Here's how the part is built. I have some questions about the finished solid (model axes, mm). Face numbers are marked on the shaded views. A direction names the side the tool comes from. Give positions to 0.01 mm unless a question says otherwise; leave off trailing zeros. Loops run counter-clockwise (first coordinate to the right, second up) from the corner with the lowest first, then second, coordinate; pieces in that order, holes last. Notation, with made-up numbers: (76, 43.5) - (87, 43.5) arc R10 ccw to (87, 49.5) - close; hole circle Ø3 at (-24, -22.5). An arc over 180 degrees is marked (long way). Return JSON: item names as keys, results as strings. Group by question number.
(1) On a 3-axis mill with a long thin cutter (end or side, diameter ignored), from which of +Z, -Z, +X, -X, +Y, -Y can I reach the whole of each face in a straight line? I mean the marked faces 1 and 2. Say none if no direction works.
(2) If we section it at A-A (z = -3.25): Please give me the cut outline in (x, y), then the cut area to 3 significant figures.
(3) If we mould it in two halves opening along Y, with no side actions, what happens to the marked faces 3, 4, 5 and 6? For each: released by +Y, released by -Y, zero draft, split by the parting line, or undercut.
(4) If we section it at B-B (y = -4): Please give me the cut outline in (x, z).
(5) If we section it at C-C (x = 17): Please give me the cut outline in (y, z), then the cut area to 3 significant figures.
(6) I need wall thicknesses on probe 1 along Z at (x, y) = (0, -5.75); probe 2 along Y at (x, z) = (17, 8); probe 3 along X at (y, z) = (-4.75, -7.5). Which ranges of each line are inside material? Lowest first, please. Write a range as [from, to].
(7) If we section it at D-D (z = 7.5): Please give me the cut outline in (x, y), then the cut area to 3 significant figures.
(8) For P1, Ø5, axis at x = -16.5, z = -7.5, coming from the +Y side; P2, Ø4, axis at x = -4.5, y = -4.5, coming from the -Z side, each with a flat end and sliding along its axis, tell me the tip position at first contact or that it passes through.
```python
from build123d import *

# Parameters (mm, degrees)
F0_R     = 3
F0_R_2   = 4
F1_DEPTH = 8
F2_R     = 2.25
F3_DEPTH = 28.001


with BuildPart() as f1:
    # F0 (on Front) → F1 (new body)
    with BuildSketch(Plane.XZ):
        Polygon((21, 14), (-21, 14), (-21, -14), (-13, -14), (-13, -2), (13, -2), (13, -14), (21, -14), align=None)
        with Locations((-10, 9)):
            Circle(F0_R, mode=Mode.SUBTRACT)
        with Locations((0, 7)):
            Circle(F0_R_2, mode=Mode.SUBTRACT)
        with Locations((10, 9)):
            Circle(F0_R, mode=Mode.SUBTRACT)
    extrude(amount=F1_DEPTH)

    # F2 (on face) → F3 (cut, through all)
    with BuildSketch(Plane.XY.offset(14)):
        with Locations((-17, -4)):
            Circle(F2_R)
        with Locations((17, -4)):
            Circle(F2_R)
    extrude(amount=-F3_DEPTH, mode=Mode.SUBTRACT)


solid = f1.part
```
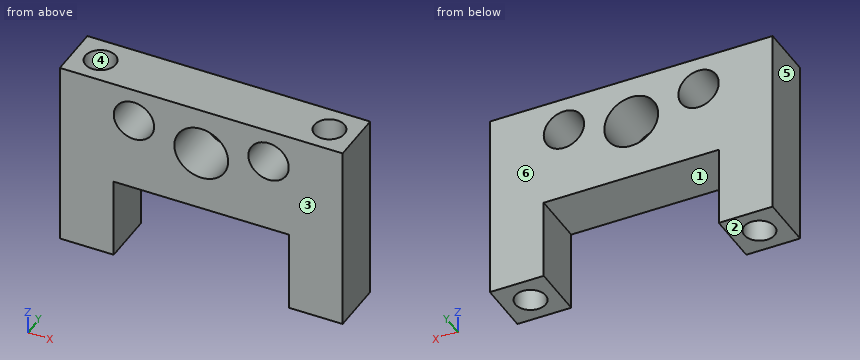
Values:
{
 "1": {"face 1": "-Z, +Y, -Y", "face 2": "-Z, +X, -X, +Y, -Y"},
 "2": {"outline": "(-21, -8) - (-13, -8) - (-13, 0) - (-21, 0) - close; (13, -8) - (21, -8) - (21, 0) - (13, 0) - close; hole circle Ø4.5 at (-17, -4); hole circle Ø4.5 at (17, -4)", "area": "96.2 mm2"},
 "3": {"face 3": "released by -Y", "face 4": "undercut", "face 5": "zero draft", "face 6": "released by +Y"},
 "4": {"outline": "(-21, -14) - (-19.25, -14) - (-19.25, 14) - (-21, 14) - close; (-14.75, -14) - (-13, -14) - (-13, -2) - (13, -2) - (13, -14) - (14.75, -14) - (14.75, 14) - (-14.75, 14) - close; (19.25, -14) - (21, -14) - (21, 14) - (19.25, 14) - close; hole circle Ø6 at (-10, 9); hole circle Ø8 at (0, 7); hole circle Ø6 at (10, 9)"},
 "5": {"outline": "(-8, -14) - (-6.25, -14) - (-6.25, 14) - (-8, 14) - close; (-1.75, -14) - (0, -14) - (0, 14) - (-1.75, 14) - close", "area": "98.0 mm2"},
 "6": {"probe 1": "[-2, 3], [11, 14]", "probe 2": "[-8, -6.25], [-1.75, 0]", "probe 3": "[-21, -19.12], [-14.88, -13], [13, 14.88], [19.12, 21]"},
 "7": {"outline": "(-21, -8) - (-12.6, -8) - (-12.6, 0) - (-21, 0) - close; (-7.4, -8) - (-3.97, -8) - (-3.97, 0) - (-7.4, 0) - close; (3.97, -8) - (7.4, -8) - (7.4, 0) - (3.97, 0) - close; (12.6, -8) - (21, -8) - (21, 0) - (12.6, 0) - close; hole circle Ø4.5 at (-17, -4); hole circle Ø4.5 at (17, -4)", "area": "158 mm2"},
 "8": {"P1": "y = 0", "P2": "z = -2"}
}
